```python
from build123d import *

# Parameters (mm, degrees)
F2_DEPTH = 10
F4_D     = 5.4


# Not quite as in the source:
# - a feature names something its author has since deleted; it is built from what else it names


with BuildPart() as f2:
    # F1 (on Front) → F2 (new body)
    with BuildSketch(Plane.XZ):
        Polygon((-36.8737237304, 13.780983012), (-63.8737237304, 13.780983012), (-63.8737237304, -22.219016988), (-36.8737237304, -22.219016988), (-36.8737237304, -52.219016988), (-26.8737237304, -52.219016988), (-26.8737237304, -12.219016988), (-36.8737237304, -12.219016988), (-53.7737237304, -12.219016988), (-53.7737237304, 3.780983012), (-36.8737237304, 3.780983012), align=None)
    extrude(amount=F2_DEPTH)

    # F4 (through all)
    with Locations(Plane.XY.offset(13.780983012)):
        with Locations((-50.3737237304, -5)):
            Hole(F4_D / 2)


solid = f2.part
```
Could you check a few things on this model? Use its own coordinates, in mm. A direction names the side the tool comes from. Give positions to 0.01 mm unless a question says otherwise; leave off trailing zeros. Write each loop counter-clockwise with the first axis right and the second up, starting at its lowest first coordinate (ties: lowest second). Pieces come first, ordered by that corner, then holes. Notation, with made-up numbers: (40.25, -21) - (96.25, -21) arc R7 cw to (96.25, -8) - close; hole circle Ø10 at (54, 26). An arc over 180 degrees is marked (long way). One line per item, written item: value. Start each with the question number.
Item 1: Imagine slicing it at D-D, the plane x = -59.5. List the corners of the cut face in (y, z) for me, and give its area (3 significant figures).
Item 2: Which directions (+Z, -Z, +X, -X, +Y, -Y) give clear straight access to the entire face, cutting with the end or side of a thin tool? Please do faces 4 (the face through (-40, -5, -12.219)), 5 (the face through (-47.676, -4.881, 8.711)), 6 (the face through (-36.874, -5, 9)), 7 (the face through (-54, -5, -22.219)), 8 (the face through (-46, -10, -19)).
Item 3: Imagine slicing it at A-A, the plane x = -46. List the corners of the cut face in (y, z) for me.
Item 4: Imagine slicing it at B-B, the plane y = -5. List the corners of the cut face in (x, z) for me, and give its area (3 significant figures).
Item 5: If we mould it in two halves opening along Y, with no side actions, what happens to faces 1 (the face through (-26.874, -5, -32)), 2 (the face through (-46, 0, -19)), 3 (the face through (-47.676, -4.881, -17.289))? For each: +Y half, -Y half, draft (parallel to the pull), parting line (faces both ways), or undercut.
Item 6: Imagine slicing it at C-C, the plane z = -13. List the corners of the cut face in (x, y) for me.
Item 7: Please list where these lines run through material, in increasing order: line 1 (Z direction, x = -42.5, y = -7.5); line 2 (X direction, y = -9.25, z = 8.5); line 3 (X direction, y = -7.5, z = -27.5). Write a range as from..to.
Item 8: I'm going to push flat-ended pins straight in: pin 1 (1 mm diameter, centred on x = -46.5, y = -7.5, fed in from -Z); pin 2 (3 mm diameter, centred on y = -5.5, z = -3, fed in from +X); pin 3 (5 mm diameter, centred on x = -50.37, y = -5, fed in from +Z); pin 4 (5 mm diameter, centred on y = -3.5, z = -42, fed in from -X). Where does each tip first touch, or does it pass through?
Geometry says:
1. outline: (-10, -22.22) - (0, -22.22) - (0, 13.78) - (-10, 13.78) - close
1. area: 360 mm^2
2. face 4: +X, +Y, -Y
2. face 5: +Z, -Z
2. face 6: +Z, +X, +Y, -Y
2. face 7: -Z, -X, +Y, -Y
2. face 8: +Z, -Z, +X, -X, -Y
3. outline: (-10, -22.22) - (0, -22.22) - (0, -12.22) - (-10, -12.22) - close; (-10, 3.78) - (0, 3.78) - (0, 13.78) - (-10, 13.78) - close
4. outline: (-63.87, -22.22) - (-53.07, -22.22) - (-53.07, -12.22) - (-53.77, -12.22) - (-53.77, 3.78) - (-53.07, 3.78) - (-53.07, 13.78) - (-63.87, 13.78) - close; (-47.67, -22.22) - (-36.87, -22.22) - (-36.87, -52.22) - (-26.87, -52.22) - (-26.87, -12.22) - (-47.67, -12.22) - close; (-47.67, 3.78) - (-36.87, 3.78) - (-36.87, 13.78) - (-47.67, 13.78) - close
4. area: 994 mm^2
5. face 1: draft
5. face 2: +Y half
5. face 3: undercut
6. outline: (-63.87, -10) - (-26.87, -10) - (-26.87, 0) - (-63.87, 0) - close; hole circle Ø5.4 at (-50.37, -5)
7. line 1: -22.22..-12.22, 3.78..13.78
7. line 2: -63.87..-36.87
7. line 3: -36.87..-26.87
8. pin 1: z = -22.22
8. pin 2: x = -53.77
8. pin 3: through
8. pin 4: x = -36.87
